Verification items for the finished model (mm, model axes). Give positions to 0.01 mm unless a question says otherwise; leave off trailing zeros. Loops run counter-clockwise (first coordinate to the right, second up) from the corner with the lowest first, then second, coordinate; pieces in that order, holes last. Notation, with made-up numbers: M 60.5,83 L 110.5,83 A14 cw 110.5,106 Z; hole C -5.75,18.25 d4. An arc over 180 degrees is marked long. Answer in a Markdown table with one row per item.
```python
from build123d import *

# Parameters (mm, degrees)
SKETCH1_W           = 8
SKETCH1_H           = 8
SKETCH1_R           = 1.5
BOSS_EXTRUDE1_DEPTH = 71.54
CUT_EXTRUDE1_REACH  = 74.097
SKETCH2_R           = 2


with BuildPart() as part:
    # Sketch1 → Boss-Extrude1 (new body)
    with BuildSketch(Plane(origin=(0, 0, 0), x_dir=(1, 0, 0), z_dir=(0, 1, 0))):
        Rectangle(SKETCH1_W, SKETCH1_H)
        with Locations(Location((0, 0, 0), (0, 0, 270))):
            Circle(SKETCH1_R, mode=Mode.SUBTRACT)
    extrude(amount=BOSS_EXTRUDE1_DEPTH)

    # Sketch2 → Cut-Extrude1 (cut, up to next)
    with BuildSketch(Plane(origin=(4, 0, 0), x_dir=(0, 0, -1), z_dir=(1, 0, 0)), mode=Mode.PRIVATE) as cut_extrude1_sk1:
        with Locations((0, 35.77)):
            Circle(SKETCH2_R)
    cut_extrude1_tool1 = extrude(cut_extrude1_sk1.sketch, amount=-CUT_EXTRUDE1_REACH, mode=Mode.PRIVATE) & part.part
    add(cut_extrude1_tool1.solids().sort_by_distance((4, 35.77, 0))[0], mode=Mode.SUBTRACT)


solid = part.part
```
Item 1: Sectioned sample at A-A (y = 35.77). Record the cut outline in (x, z).
Reported:
| item | result |
|---|---|
| outline | M -4,-4 L 4,-4 L 4,-2 L -4,-2 Z; M -4,2 L 4,2 L 4,4 L -4,4 Z |
Item 2: Sectioned sample at C-C (x = 0). Record the cut outline in (y, z).
Reported:
| item | result |
|---|---|
| outline | M 0,-4 L 71.54,-4 L 71.54,-1.5 L 37.09,-1.5 A2 cw 34.45,-1.5 L 0,-1.5 Z; M 0,1.5 L 34.45,1.5 A2 cw 37.09,1.5 L 71.54,1.5 L 71.54,4 L 0,4 Z |
Item 3: Go/stop test with a flat-tipped pin: pin 1 (4 mm diameter, centred on x = 0, z = 0, fed in from +Y). Record where the tip stops, or that it passes through.
Reported:
| item | result |
|---|---|
| pin 1 | stops at y = 71.54 |
Item 4: Sectioned sample at B-B (z = 0). Record the cut outline in (x, y), and give its area (3 significant figures).
Reported:
| item | result |
|---|---|
| outline | M -4,0 L -1.5,0 L -1.5,33.77 L -4,33.77 Z; M -4,37.77 L -1.5,37.77 L -1.5,71.54 L -4,71.54 Z; M 1.5,0 L 4,0 L 4,33.77 L 1.5,33.77 Z; M 1.5,37.77 L 4,37.77 L 4,71.54 L 1.5,71.54 Z |
| area | 338 mm^2 |
Item 5: Release check for a two-part mould opening along Z. For faces 1 (the flat face through (0, 35, -4)), 2 (the flat face through (-4, 35, 3)), 3 (the cylindrical face through (0.45, 16.98, 1.43)), 4 (the flat face through (0, 35, 4)) record: released by +Z, released by -Z, zero draft, split by the parting line, or undercut.
Reported:
| item | result |
|---|---|
| face 1 | released by -Z |
| face 2 | zero draft |
| face 3 | undercut |
| face 4 | released by +Z |
Item 6: Sectioned sample at D-D (y = 57). Record the cut outline in (x, z), and give its area (3 significant figures).
Reported:
| item | result |
|---|---|
| outline | M -4,-4 L 4,-4 L 4,4 L -4,4 Z; hole C 0,0 d3 |
| area | 56.9 mm^2 |
Item 7: Scan lines: L1, parallel to Z at x = 0, y = 27.5; L2, parallel to Y at x = 3, z = 0.75. Record each from-to range of solid material in increasing order. Write a range as [from, to].
Reported:
| item | result |
|---|---|
| L1 | z = [-4, -1.5], [1.5, 4] |
| L2 | y = [0, 33.92], [37.62, 71.54] |
